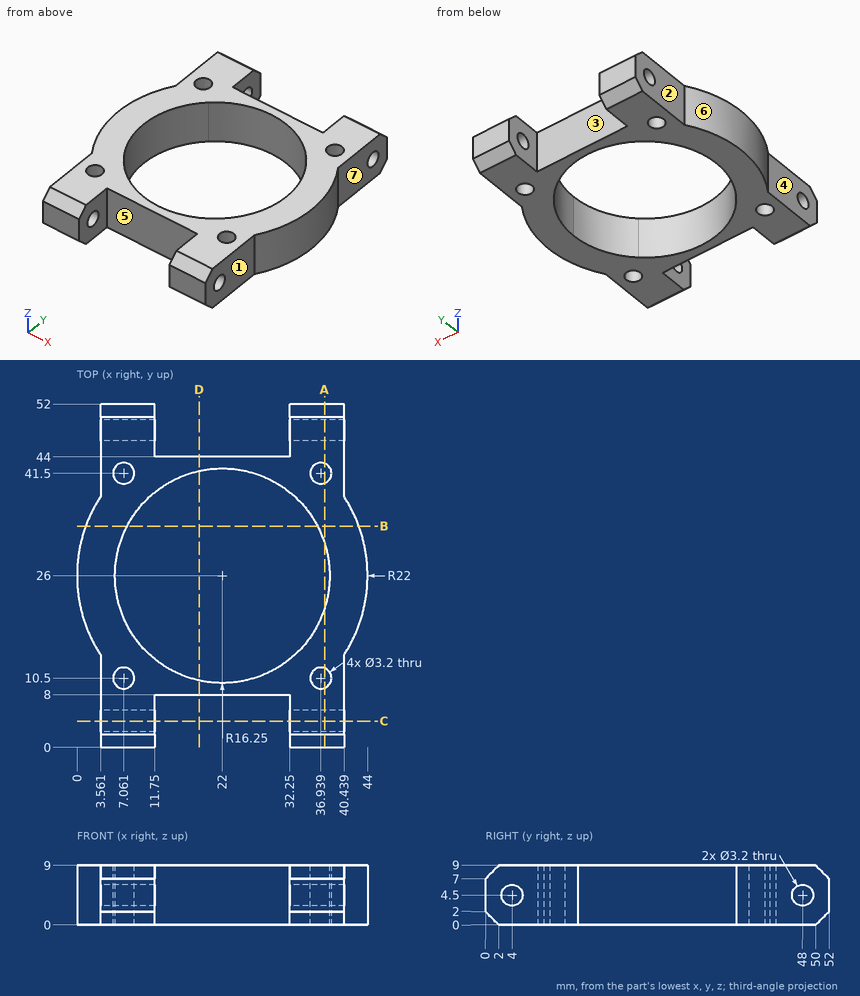
Can you work these out from the drawing? Everything is in mm from the part's minimum corner. A direction names the side the tool comes from. Round coordinates to 2 decimals unless told otherwise and drop trailing zeros. Loops run counter-clockwise (first coordinate to the right, second up) from the corner with the lowest first, then second, coordinate; pieces in that order, holes last. Notation, with made-up numbers: (-16.75, 25.5) -> (29.25, 25.5) arc R24 ccw to (29.25, 64.5) -> close; hole circle Ø11 at (68.25, 27). An arc over 180 degrees is marked (long way). Use CSV: the item, a comma, the result in double quotes.
(1) Suppose I cut it at C-C on y = 4. Write out the boundary of the cut face in (x, z), plus the area to 3 significant figures.
Return value:
outline,"(3.56, 0) -> (11.75, 0) -> (11.75, 2.9) -> (3.56, 2.9) -> close; (3.56, 6.1) -> (11.75, 6.1) -> (11.75, 9) -> (3.56, 9) -> close; (32.25, 0) -> (40.44, 0) -> (40.44, 2.9) -> (32.25, 2.9) -> close; (32.25, 6.1) -> (40.44, 6.1) -> (40.44, 9) -> (32.25, 9) -> close"
area,"95.0 mm²"
(2) Suppose I cut it at A-A on x = 37.5. Write out the boundary of the cut face in (y, z).
Return value:
outline,"(0, 2) -> (2, 0) -> (9, 0) -> (9, 9) -> (2, 9) -> (0, 7) -> close; (12, 0) -> (21.12, 0) -> (21.12, 9) -> (12, 9) -> close; (30.88, 0) -> (40, 0) -> (40, 9) -> (30.88, 9) -> close; (43, 0) -> (50, 0) -> (52, 2) -> (52, 7) -> (50, 9) -> (43, 9) -> close; hole circle Ø3.2 at (4, 4.5); hole circle Ø3.2 at (48, 4.5)"
(3) Will these pins go through, and if not, where does the flat tip stop? pin 1 Ø3 at (x, y) = (36.94, 41.5) entering from +Z; pin 2 Ø2 at (y, z) = (41, 2) entering from +X; pin 3 Ø1 at (x, z) = (18, 6.5) entering from +Y; pin 4 Ø2.5 at (y, z) = (43, 5) entering from -X.
Return value:
pin 1,"passes through"
pin 2,"stops at x = 40.44"
pin 3,"stops at y = 44"
pin 4,"stops at x = 3.56"
(4) Suppose I cut it at B-B on y = 33.5. Write out the boundary of the cut face in (x, z).
Return value:
outline,"(1.32, 0) -> (7.58, 0) -> (7.58, 9) -> (1.32, 9) -> close; (36.42, 0) -> (42.68, 0) -> (42.68, 9) -> (36.42, 9) -> close"
(5) For the marked faces 1, 2, 3 and 4, which set-ups out of +Z, -Z, +X, -X, +Y, -Y let a thin tool reach every point of the face, with its end or its side?
Return value:
face 1,"+Z, -Z, +X, -Y"
face 2,"+Z, -Z, -X, +Y"
face 3,"+Z, -Z, +Y"
face 4,"+Z, -Z, -X, -Y"
(6) Suppose I cut it at D-D on x = 18.5. Write out the boundary of the cut face in (y, z).
Return value:
outline,"(8, 0) -> (10.13, 0) -> (10.13, 9) -> (8, 9) -> close; (41.87, 0) -> (44, 0) -> (44, 9) -> (41.87, 9) -> close"
(7) If I drill on probe 1 along X at (y, z) = (5, 2); probe 2 along Z at (x, y) = (37.5, 4); probe 3 along X at (y, z) = (41, 6.5), over which ranges is the centre line in solid material (lowest first)? Write a range as [from, to].
Return value:
probe 1,"x = [3.56, 11.75], [32.25, 40.44]"
probe 2,"z = [0, 2.9], [6.1, 9]"
probe 3,"x = [3.56, 5.54], [8.58, 15.75], [28.25, 35.42], [38.46, 40.44]"
(8) If we mould it in two halves opening along X, with no side actions, what happens to the marked faces 5, 6 and 7? For each: +X half, -X half, draft (parallel to the pull), parting line (faces both ways), or undercut.
Return value:
face 5,"undercut"
face 6,"-X half"
face 7,"+X half"
